Autodesk Inventor part; units mm, degrees
ref_plane "YZ Plane" through (0, 0, 0) normal (1, 0, 0) x (0, 1, 0)
ref_plane "XZ Plane" through (0, 0, 0) normal (0, 1, 0) x (-1, 0, 0)
ref_plane "XY Plane" through (0, 0, 0) normal (0, 0, 1) x (1, 0, 0)
sketch "スケッチ1" plane through (0, 0, 0) normal (0, 1, 0) x (-1, 0, 0)
  line L0 (-2, 0) -> (-2, 2.8)
  line L1 (-2, 2.8) -> (-2.75, 2.8)
  line L2 (-2.75, 2.8) -> (-2.75, 2.3)
  line L3 (-2.75, 2.3) -> (-4.0415, 2.3)
  line L4 (-4.0415, 2.3) -> (-4.0415, 0.3126)
  line L5 (-3.5, 0) -> (-2, 0)
  line L6 (-4.0415, 0.3126) -> (-3.5, 0)
  line L7 (0, -0.56) -> (0, 3.36)
  point P0 (0, 0)
  dimension "d0" = 3.5
  dimension "d1" = 4.0415
  dimension "d2" = 30
  dimension "d3" = 0.5
  dimension "d4" = 2.8
  dimension "d5" = 4
  dimension "d6" = 5.5
revolve "回転1" add sketch "スケッチ1" angle 360 about axis through (0, 0, -10) along (0, 0, 1)
sketch "スケッチ2" plane through (0, 0, 0) normal (0, 0, -1) x (-1, 0, 0)
  circle A0 centre (0, 0) radius 4.0415
  line L0 (0, 4.0415) -> (3.5, 2.0207)
  line L1 (3.5, 2.0207) -> (3.5, -2.0207)
  line L2 (3.5, -2.0207) -> (0, -4.0415)
  line L3 (0, -4.0415) -> (-3.5, -2.0207)
  line L4 (-3.5, -2.0207) -> (-3.5, 2.0207)
  line L5 (-3.5, 2.0207) -> (0, 4.0415)
  point P0 (-3.5, 2.0207)
  point P1 (-3.5, 2.0207)
  point P2 (-3.5, -2.0207)
  point P3 (-3.5, -2.0207)
  point P4 (0, -4.0415)
  point P5 (0, -4.0415)
  point P6 (3.5, -2.0207)
  point P7 (3.5, -2.0207)
  point P8 (3.5, 2.0207)
  point P9 (3.5, 2.0207)
extrude "押し出し1" cut sketch "スケッチ2" against normal through all contours A0 L1 | L0 A0 | A0 L2 | L5 A0 | A0 L3 | L4 A0
chamfer "面取り1" distance 0.3 angle 45 6 edges at (0, 4.0415, 1.3063) (-3.5, 2.0207, 1.3063) (3.5, 2.0207, 1.3063) (3.5, -2.0207, 1.3063) (0, -4.0415, 1.3063) (-3.5, -2.0207, 1.3063)
thread "ねじ1"
properties part number "S4-05-3W" material "チタン"
Verification items for the finished model (mm, model axes). A direction names the side the tool comes from. Round coordinates to 2 decimals unless told otherwise and drop trailing zeros. Write each loop counter-clockwise with the first axis right and the second up, starting at its lowest first coordinate (ties: lowest second). Pieces come first, ordered by that corner, then holes. Notation, with made-up numbers: (9.5, -12) - (16.5, -12) arc R28 ccw to (16.5, 8) - close; hole circle Ø9 at (50, 24). An arc over 180 degrees is marked (long way). Answer as a JSON object with one key per item and string values. Group by question number.
Q1. Tool access check on faces 1 (the flat face through (-1, -3, 2.3)), 2 (the flat face through (-3.5, 0, 1)). Record the directions out of +Z, -Z, +X, -X, +Y, -Y that give a thin tool (end or side, any length) a straight path to the whole face; none if there is none.
Q2. Section check A-A, the plane x = 0. Enter the section's corners in (y, z).
Q3. Section check B-B, the plane z = 0.85. Enter the section's corners in (x, y).
Q4. Thickness scan on line 1 (Y direction, x = 0, z = 1); line 2 (Z direction, x = 1, y = 3); line 3 (X direction, y = -0.25, z = 2). Record the ranges inside material, lowest first.
Q5. Mould release check, pull along X, two halves, no side actions. Record for faces 3 (the cylindrical face through (0, -2, 1)), 4 (the conical face through (-3.15, 1.85, 0.09)), 5 (the flat face through (2, -2, 0)): released by +X, released by -X, zero draft, split by the parting line, or undercut.
Found:
{
 "1": {"face 1": "+Z", "face 2": "+Z, -Z, -X, +Y, -Y"},
 "2": {"outline": "(-3.89, 0.23) - (-3.5, 0) - (-2, 0) - (-2, 2.8) - (-2.75, 2.8) - (-2.75, 2.3) - (-3.89, 2.3) - close; (2, 0) - (3.5, 0) - (3.89, 0.23) - (3.89, 2.3) - (2.75, 2.3) - (2.75, 2.8) - (2, 2.8) - close"},
 "3": {"outline": "(-3.5, -1.72) - (-3.24, -2.17) - (-0.26, -3.89) - (0.26, -3.89) - (3.24, -2.17) - (3.5, -1.72) - (3.5, 1.72) - (3.24, 2.17) - (0.26, 3.89) - (-0.26, 3.89) - (-3.24, 2.17) - (-3.5, 1.72) - close; hole circle Ø4 at (0, 0)"},
 "4": {"line 1": "y = -3.89 to -2, 2 to 3.89", "line 2": "z = 0 to 2.3", "line 3": "x = -3.5 to -1.98, 1.98 to 3.5"},
 "5": {"face 3": "undercut", "face 4": "released by -X", "face 5": "zero draft"}
}
